Read the model definition and answer for the solid it produces. Units are mm, in the model's axes. Coordinates: 2 decimals unless noted, no trailing zeros. Write each loop counter-clockwise with the first axis right and the second up, starting at its lowest first coordinate (ties: lowest second). Pieces come first, ordered by that corner, then holes. Notation, with made-up numbers: (43, 48) -> (81, 48) arc R19 ccw to (81, 67) -> close; hole circle Ø4 at (39.5, -36.75). An arc over 180 degrees is marked (long way). Answer as a JSON object with one key per item and string values. Group by question number.
(1) Find section B-B (z = -4.5). Give the vertices of the cut face in (x, y), then the cut area to 3 significant figures.
(2) Straight lines are drawn through the part: L1, parallel to Z at x = -3.75, y = -18.5; L2, parallel to Z at x = 4.25, y = -24.5. For each, find the intervals that lie inside material, in ascending order.
(3) A flat-ended cylindrical pin translates along its axis: P1, Ø2, axis at x = -1.5, y = -21.5, coming from the +Z side. Find the tip coordinate at first contact, or state that the pin passes through.
(4) Find section C-C (y = -20). Give the vertices of the cut face in (x, z), then the cut area to 3 significant figures.
(5) Find section A-A (x = -0.5). Give the vertices of the cut face in (y, z).
from build123d import *

# Parameters (mm, degrees)
PLAT_W                       = 55
PLAT_H                       = 10
EL_MENT_M_CANO_SOUD_1_DEPTH  = 10
ENL_V_MAT_EXTRU_1_DEPTH      = 6
ENL_V_MAT_EXTRU_1_DEPTH_BACK = 6


with BuildPart() as part:
    # plat → Elément mécano-soudé1 (new body)
    with BuildSketch(Plane.YZ.offset(-5)):
        Rectangle(PLAT_W, PLAT_H)
    extrude(amount=EL_MENT_M_CANO_SOUD_1_DEPTH)

    # Esquisse2 → Enlèv. mat.-Extru.1 (cut, two sides)
    with BuildSketch(Plane(origin=(0, 0, 0), x_dir=(0, 0, -1), z_dir=(1, 0, 0))) as enl_v_mat_extru_1_sk:
        Polygon((-3, -27.5), (-5, -18.478582993), (-5, -27.5), align=None)
        Polygon((5, -27.5), (5, -18.478582993), (3, -27.5), align=None)
    extrude(amount=ENL_V_MAT_EXTRU_1_DEPTH, mode=Mode.SUBTRACT)
    extrude(enl_v_mat_extru_1_sk.sketch, amount=-ENL_V_MAT_EXTRU_1_DEPTH_BACK, mode=Mode.SUBTRACT)


solid = part.part
Results below:
{
 "1": {"outline": "(-5, -20.73) -> (5, -20.73) -> (5, 27.5) -> (-5, 27.5) -> close", "area": "482 mm2"},
 "2": {"L1": "z = -5 to 5", "L2": "z = -3.67 to 3.67"},
 "3": {"P1": "stops at z = 4.55"},
 "4": {"outline": "(-5, -4.66) -> (5, -4.66) -> (5, 4.66) -> (-5, 4.66) -> close", "area": "93.3 mm2"},
 "5": {"outline": "(-27.5, -3) -> (-18.48, -5) -> (27.5, -5) -> (27.5, 5) -> (-18.48, 5) -> (-27.5, 3) -> close"}
}
